The drawing under review shows one solid part. Ordinate dimensions are in mm from its lowest x, y, z. A direction names the side the tool comes from. Coordinates: 2 decimals unless noted, no trailing zeros. Loops run counter-clockwise (first coordinate to the right, second up) from the corner with the lowest first, then second, coordinate; pieces in that order, holes last. Notation, with made-up numbers: (-35.5, -3.5) -> (-22.5, -3.5) arc R19 cw to (-22.5, 17.5) -> close; hole circle Ø11 at (17.25, -0.5). An arc over 180 degrees is marked (long way). Use a Markdown table: item, result.
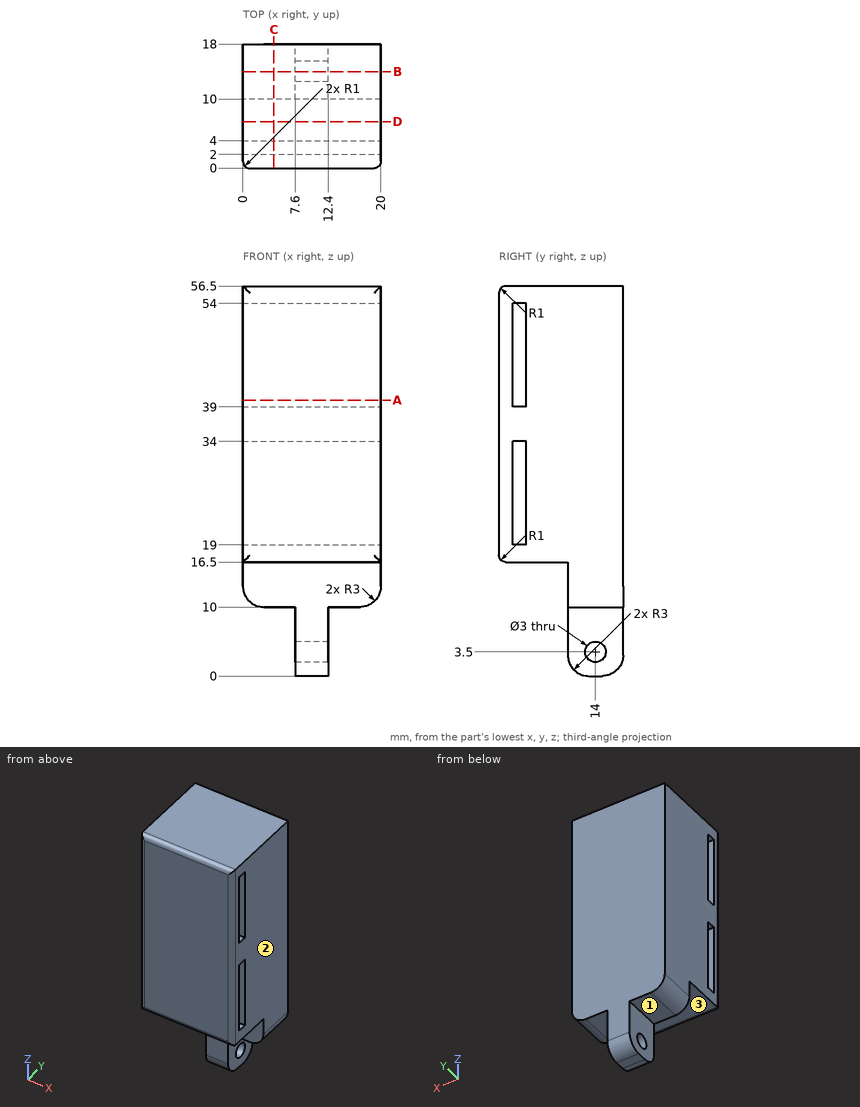
(1) For pin 1 Ø2.5 at (y, z) = (14, 3.5) entering from +X; pin 2 Ø4 at (x, z) = (9.5, 12.5) entering from -Y; pin 3 Ø1.4 at (x, y) = (5, 13) entering from -Z; pin 4 Ø6.5 at (y, z) = (16, 2.5) entering from +X, all flat-tipped, find the tip position at first contact; note any pin that passes through.
Found:
| item | result |
|---|---|
| pin 1 | passes through |
| pin 2 | stops at y = 10 |
| pin 3 | stops at z = 10 |
| pin 4 | stops at x = 12.4 |
(2) Take a section at B-B on y = 14. Write out the cut boundary in (x, z).
Found:
| item | result |
|---|---|
| outline | (0, 13) arc R3 ccw to (3, 10) -> (7.6, 10) -> (7.6, 5) -> (12.4, 5) -> (12.4, 10) -> (17, 10) arc R3 ccw to (20, 13) -> (20, 56.5) -> (0, 56.5) -> close; (7.6, 0) -> (12.4, 0) -> (12.4, 2) -> (7.6, 2) -> close |
(3) For line 1 along Z through (x, y) = (10, 14); line 2 along Y through (x, z) = (11, 41.5); line 3 along Y through (x, z) = (10.55, 3.5), list the stretches that pass through material, from the lowest coordinate up.
Found:
| item | result |
|---|---|
| line 1 | z = 0 to 2, 5 to 56.5 |
| line 2 | y = 0 to 2, 4 to 18 |
| line 3 | y = 10 to 12.5, 15.5 to 18 |
(4) Take a section at D-D on y = 6.75. Write out the cut boundary in (x, z).
Found:
| item | result |
|---|---|
| outline | (0, 16.5) -> (20, 16.5) -> (20, 56.5) -> (0, 56.5) -> close |
(5) Take a section at C-C on x = 4.5. Write out the cut boundary in (y, z).
Found:
| item | result |
|---|---|
| outline | (0, 17.5) arc R1 ccw to (1, 16.5) -> (10, 16.5) -> (10, 10) -> (18, 10) -> (18, 56.5) -> (1, 56.5) arc R1 ccw to (0, 55.5) -> close; hole (2, 19) -> (4, 19) -> (4, 34) -> (2, 34) -> close; hole (2, 39) -> (4, 39) -> (4, 54) -> (2, 54) -> close |
(6) For the marked faces 1, 2 and 3, list the 3-axis set-ups (+Z, -Z, +X, -X, +Y, -Y) from which the entire face can be reached by the end or side of a thin tool; tool diameter is ignored.
Found:
| item | result |
|---|---|
| face 1 | -Z, -X, +Y, -Y |
| face 2 | +Z, -Z, +X, +Y, -Y |
| face 3 | -Z, +X, -X, -Y |
(7) Take a section at A-A on z = 40. Write out the cut boundary in (x, y).
Found:
| item | result |
|---|---|
| outline | (0, 1) arc R1 ccw to (1, 0) -> (19, 0) arc R1 ccw to (20, 1) -> (20, 2) -> (0, 2) -> close; (0, 4) -> (20, 4) -> (20, 18) -> (0, 18) -> close |
